from build123d import *

# Parameters (mm, degrees)
EXTRUDE_1_DEPTH         = 1.52
CUT_EXTRUDE_START       = -3
CUT_EXTRUDE_1_OUTLINE_W = 7
CUT_EXTRUDE_1_OUTLINE_H = 2.04
CUT_EXTRUDE_1_DEPTH     = 3


# Read off the part's stored shape, not the designer's step: Вырез-Вытянуть1
with BuildPart() as part:
    # Эскиз1 → Повернуть1 (revolve)
    with BuildSketch(Plane(origin=(0, 0, 0), x_dir=(0, 0, -1), z_dir=(1, 0, 0)), mode=Mode.PRIVATE) as revolve_1_sk:
        with BuildLine():
            Line((-2.5, 1), (0, 1))
            Line((0, 1), (0, 8.7))
            ThreePointArc((0, 8.7), (-1.767766953, 7.967766953), (-2.5, 6.2))
            Line((-2.5, 6.2), (-2.5, 1))
        make_face()
        Polygon((-3.25, 1), (-3.25, 0), (0, 0), (0, 1), (-2.5, 1), align=None)
    revolve(revolve_1_sk.sketch.rotate(Axis((0, -2.603301624, 0), (0, 1, 0)), 180), axis=Axis((0, -2.603301624, 0), (0, 1, 0)))

    # Эскиз2 → Бобышка-Вытянуть1 (add, symmetric)
    with BuildSketch(Plane.XY):
        with BuildLine():
            Line((0.25, 0), (0.25, -1.5))
            ThreePointArc((0.25, -1.5), (-0.189339828, -2.560660172), (-1.25, -3))
            Line((-1.25, -3), (-6.75, -3))
            Line((-6.75, -3), (-6.75, -2.5))
            Line((-6.75, -2.5), (-1.75, -2.5))
            ThreePointArc((-1.75, -2.5), (-0.689339828, -2.060660172), (-0.25, -1))
            Line((-0.25, -1), (-0.25, 0))
            Line((-0.25, 0), (0.25, 0))
        make_face()
    extrude(amount=EXTRUDE_1_DEPTH, both=True)

    # Вырез-Вытянуть1 outline → Вырез-Вытянуть1 (cut)
    with BuildSketch(Plane.XZ.offset(3).offset(CUT_EXTRUDE_START)):
        with Locations((-3.25, 0)):
            Rectangle(CUT_EXTRUDE_1_OUTLINE_W, CUT_EXTRUDE_1_OUTLINE_H)
    extrude(amount=CUT_EXTRUDE_1_DEPTH, mode=Mode.SUBTRACT)


solid = part.part
Geometry check sheet. Reference: the model listing, model coordinates, mm. A direction names the side the tool comes from. Coordinates: 2 decimals unless noted, no trailing zeros. Order: outer loops, then holes, each group sorted by start corner. A loop starts at its lowest first (then second) coordinate and runs counter-clockwise, first axis right, second up. Notation, with made-up numbers: (71, -39) -> (79, -39) arc R26 ccw to (79, -24) -> close; hole circle Ø3 at (-3.5, 74.25). An arc over 180 degrees is marked (long way). Use a Markdown table: item, result. Add a question column.
1. Mould release check, pull along Z, two halves, no side actions. Record for faces 1 (the face through (-2.2, -2.7, -1.52)), 2 (the face through (-2.2, -2.7, -1.02)), 3 (the face through (-2.2, -2.7, 1.02)), 4 (the face through (2, 1, 2)): pulls with the +Z half, pulls with the -Z half, needs draft (parallel to the pull), parting line crosses it, or undercut.
2. Cross-section at C-C (z = 0). Enter the section's corners in (x, y).
3. Set-up check for faces 5 (the face through (-0.7, -2.07, -1.27)), 6 (the face through (-0.18, -2.55, -1.27)), 7 (the face through (-2.2, -2.7, 1.52)), 8 (the face through (-0.1, 3.6, 2.5)): record each of +Z, -Z, +X, -X, +Y, -Y from which the full face is reachable in a straight line by a thin tool's end or side.
4. Cross-section at D-D (x = 0.5). Enter the section's corners in (y, z), and give its area (3 significant figures).
5. Cross-section at B-B (x = -5). Enter the section's corners in (y, z), and give its area (3 significant figures).
6. Cross-section at A-A (y = -0.25). Enter the section's corners in (x, z).
7. Go/stop test with flat-tipped pins: pin 1 Ø3 at (y, z) = (7.5, 2) entering from -X; pin 2 Ø1 at (y, z) = (6, 1.5) entering from +X; pin 3 Ø1.5 at (x, z) = (-2.5, -1) entering from +Y. Record where each tip stops, or that it passes through.
8. Material ranges on L1, parallel to Y at x = -2.5, z = -1.25; L2, parallel to Y at x = -2.5, z = 2; L3, parallel to Z at x = 2, y = 5.25, recorded low to high.
Filled sheet:
| question | item | result |
|---|---|---|
| 1 | face 1 | pulls with the -Z half |
| 1 | face 2 | undercut |
| 1 | face 3 | undercut |
| 1 | face 4 | needs draft |
| 2 | outline | (-3.25, 0) -> (3.25, 0) -> (3.25, 1) -> (2.5, 1) -> (2.5, 6.2) arc R2.5 ccw to (-2.5, 6.2) -> (-2.5, 1) -> (-3.25, 1) -> close |
| 3 | face 5 | +Z, -Z, -X |
| 3 | face 6 | +Z, -Z, +X, -Y |
| 3 | face 7 | +Z, +X, -X, -Y |
| 3 | face 8 | +Y |
| 4 | outline | (0, -3.21) -> (1, -3.21) -> (1, -2.45) -> (6.2, -2.45) arc R2.45 ccw to (6.2, 2.45) -> (1, 2.45) -> (1, 3.21) -> (0, 3.21) -> close |
| 4 | area | 41.3 mm2 |
| 5 | outline | (-3, -1.52) -> (-2.5, -1.52) -> (-2.5, -1.02) -> (-3, -1.02) -> close; (-3, 1.02) -> (-2.5, 1.02) -> (-2.5, 1.52) -> (-3, 1.52) -> close |
| 5 | area | 0.500 mm2 |
| 6 | outline | (-0.25, -1.52) -> (0.25, -1.52) -> (0.25, -1.02) -> (-0.25, -1.02) -> close; (-0.25, 1.02) -> (0.25, 1.02) -> (0.25, 1.52) -> (-0.25, 1.52) -> close |
| 7 | pin 1 | x = -2.34 |
| 7 | pin 2 | x = 2.29 |
| 7 | pin 3 | y = 7.77 |
| 8 | L1 | -3 to -2.5, 0 to 1 |
| 8 | L2 | 0 to 1 |
| 8 | L3 | -1.5 to 1.5 |
